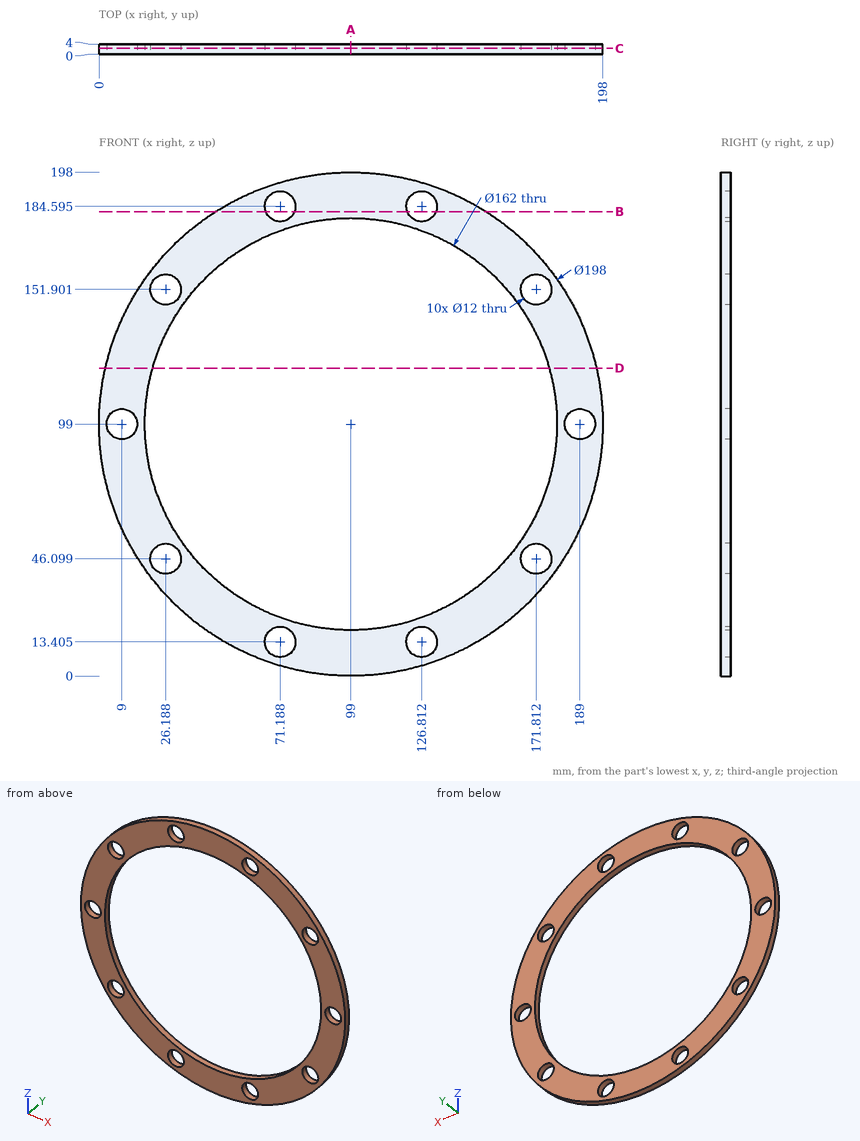
For this review, use the dimensioned drawing (mm, ordinates from the lowest corner) and the shaded views. Give positions to 0.01 mm unless a question says otherwise; leave off trailing zeros. Write each loop counter-clockwise with the first axis right and the second up, starting at its lowest first coordinate (ties: lowest second). Pieces come first, ordered by that corner, then holes.
(1) For P1, Ø1, axis at x = 40, y = 3, coming from the -Z side; P2, Ø1.5, axis at x = 107, y = 2.5, coming from the +Z side, all flat-tipped, find the tip position at first contact; note any pin that passes through.
(2) Consider section D-D, the plane z = 121. Give the boundary of the cut face in (x, y) (1 decimal).
(3) Consider section B-B, the plane z = 182.5. Give the boundary of the cut face in (x, y).
(4) Consider section C-C, the plane y = 2.25. Give the number of separate pieces and of enclosed holes in the cut face, and give its area (3 significant figures).
(5) To check wall thickness, follow L1, parallel to X at y = 1.6, z = 50.5 (1 decimal); L2, parallel to X at y = 2.05, z = 142 (1 decimal); L3, parallel to X at y = 2.9, z = 166.5 (1 decimal). State the ranges of each line that lie inside material, in increasing order.
(6) Consider section A-A, the plane x = 99. Give the boundary of the cut face in (y, z), and give its area (3 significant figures).
Returned:
1. P1: stops at z = 19.13
1. P2: stops at z = 197.73
2. outline: (2.5, 0) - (21, 0) - (21, 4) - (2.5, 4) - close; (177, 0) - (195.5, 0) - (195.5, 4) - (177, 4) - close
3. outline: (45.81, 0) - (65.57, 0) - (65.57, 4) - (45.81, 4) - close; (76.81, 0) - (121.19, 0) - (121.19, 4) - (76.81, 4) - close; (132.43, 0) - (152.19, 0) - (152.19, 4) - (132.43, 4) - close
4. separate pieces: 1
4. enclosed holes: 11
4. area: 9,050 mm2
5. L1: x = 12.7 to 22.1, 30.3 to 34.1, 163.9 to 167.7, 175.9 to 185.3
5. L2: x = 9.8 to 30.4, 167.6 to 188.2
5. L3: x = 26.6 to 54.2, 143.8 to 171.4
6. outline: (0, 0) - (4, 0) - (4, 18) - (0, 18) - close; (0, 180) - (4, 180) - (4, 198) - (0, 198) - close
6. area: 144 mm2
